Check sheet for the modelled part. Datum: model origin and axes. Units: mm. Face numbers are marked on the shaded views. A direction names the side the tool comes from. Round coordinates to 2 decimals unless told otherwise and drop trailing zeros. Order: outer loops, then holes, each group sorted by start corner. A loop starts at its lowest first (then second) coordinate and runs counter-clockwise, first axis right, second up. Notation, with made-up numbers: (-8.75, 33) -> (20.25, 33) arc R15 cw to (20.25, 46) -> close; hole circle Ø2 at (25, 35). An arc over 180 degrees is marked (long way). Answer in a Markdown table with one row per item. Add a question column.
1. Depth check by flat-ended pin: P1, Ø2.5, axis at x = 0, y = 0, coming from the -Z side; P2, Ø1.5, axis at x = 21, z = 1.5, coming from the +Y side; P3, Ø1.5, axis at y = 11.5, z = 1, coming from the +X side; P4, Ø1.5, axis at y = -10, z = 2.5, coming from the -X side. Enter the tip coordinate at first touch or a pass-through.
2. Sectioned sample at B-B, the plane y = 1. Record the boundary of the cut face in (x, z).
3. Draft check along Y on the marked faces 5, 6, 7 and 8. Enter one of: +Y half, -Y half, draft (parallel to the pull), parting line (faces both ways), or undercut.
4. Material ranges on L1, parallel to X at y = 12, z = 2.85; L2, parallel to Y at x = 17.5, z = 1.1; L3, parallel to X at y = -9, z = 0.95, recorded low to high. Write a range as from..to.
5. Access from +Z, -Z, +X, -X, +Y, -Y to the whole of each face (thin tool, end or side, straight path). Record for the marked faces 1, 2, 3 and 4.
6. Sectioned sample at D-D, the plane y = 6. Record the boundary of the cut face in (x, z), then the cut area to 3 significant figures.
7. Sectioned sample at C-C, the plane x = -7. Record the boundary of the cut face in (y, z), then the cut area to 3 significant figures.
```python
from build123d import *

# Parameters (mm, degrees)
F0_R     = 1.6
F0_W     = 6.3
F0_H     = 1
F0_W_2   = 2.5
F0_H_2   = 4
F1_DEPTH = 3
F2_R     = 2.99999
F3_R     = 6
F4_R     = 1.5


# Not quite as in the source:
# - a fillet or chamfer is up to 0.001 mm smaller than in the source, because OpenCascade refuses the exact size


with BuildPart() as f1:
    # F0 (on Top) → F1 (new body)
    with BuildSketch(Plane.XY):
        with BuildLine():
            ThreePointArc((0, 3), (-2.1213203436, 2.1213203436), (-3, 0))
            Line((-3, 0), (-3, -3))
            Line((-3, -3), (-3, -4))
            Line((-3, -4), (-9.3, -4))
            Line((-9.3, -4), (-3, -14.9119200877))
            Line((-3, -14.9119200877), (3, -14.9119200877))
            Line((3, -14.9119200877), (3, -3))
            Line((3, -3), (25, -3))
            Line((25, -3), (25, 3))
            Line((25, 3), (13, 3))
            Line((13, 3), (7, 3))
            Line((7, 3), (0, 3))
        make_face()
        Circle(F0_R, mode=Mode.SUBTRACT)
        with Locations((-6.15, -3.5)):
            Rectangle(F0_W, F0_H)
        Polygon((7, 7.5), (7, 3), (13, 3), (13, 13), (7, 13), (7, 11.5), align=None)
        with Locations((5.75, 9.5)):
            Rectangle(F0_W_2, F0_H_2)
        Polygon((7, 13), (13, 13), (13, 15.5), (6, 15.5), (6, 13), align=None)
    extrude(amount=F1_DEPTH)

    # F2 (radius 3 in the source; OpenCascade refuses exactly that, so slightly less here)
    f2_edges = [f1.edges().sort_by_distance(p)[0] for p in [
        (-3, -14.91192, 1.5),
        (3, -14.91192, 1.5),
        (25, -3, 1.5),
        (25, 3, 1.5),
        (13, 15.5, 1.5),
    ]]
    fillet(f2_edges, radius=F2_R)

    # F3
    f3_edges = [f1.edges().sort_by_distance(p)[0] for p in [
        (3, -3, 1.5),
        (13, 3, 1.5),
    ]]
    fillet(f3_edges, radius=F3_R)

    # F4
    f4_edges = [f1.edges().sort_by_distance(p)[0] for p in [
        (4.5, 11.5, 1.5),
        (4.5, 7.5, 1.5),
        (7, 3, 1.5),
    ]]
    fillet(f4_edges, radius=F4_R)


solid = f1.part
```
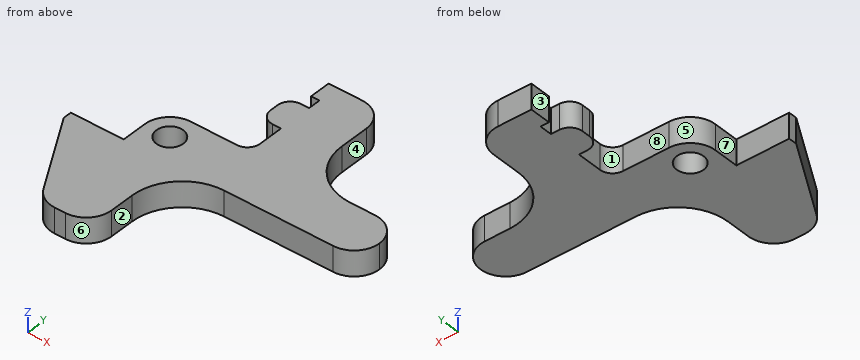
Answer key:
| question | item | result |
|---|---|---|
| 1 | P1 | passes through |
| 1 | P2 | stops at y = 3 |
| 1 | P3 | stops at x = 13 |
| 1 | P4 | stops at x = -6.27 |
| 2 | outline | (-2.83, 0) -> (-1.25, 0) -> (-1.25, 3) -> (-2.83, 3) -> close; (1.25, 0) -> (24.83, 0) -> (24.83, 3) -> (1.25, 3) -> close |
| 3 | face 5 | +Y half |
| 3 | face 6 | -Y half |
| 3 | face 7 | draft |
| 3 | face 8 | undercut |
| 4 | L1 | x = 7..13 |
| 4 | L2 | y = -3..3.19 |
| 4 | L3 | x = -6.41..3 |
| 5 | face 1 | +Z, -Z, -X |
| 5 | face 2 | +Z, -Z, +X, -Y |
| 5 | face 3 | +Z, -Z, -X, +Y |
| 5 | face 4 | +Z, -Z, +X, +Y |
| 6 | outline | (7, 0) -> (13.8, 0) -> (13.8, 3) -> (7, 3) -> close |
| 6 | area | 20.4 mm² |
| 7 | outline | (-7.98, 0) -> (-3, 0) -> (-3, 3) -> (-7.98, 3) -> close |
| 7 | area | 15.0 mm² |
